Part model, mm, in its own coordinate system. Face numbers are marked on the shaded views. Round coordinates to 2 decimals unless told otherwise and drop trailing zeros. Order: outer loops, then holes, each group sorted by start corner. A loop starts at its lowest first (then second) coordinate and runs counter-clockwise, first axis right, second up. Notation, with made-up numbers: (-31.5, 54) - (12.5, 54) arc R16 cw to (12.5, 69) - close; hole circle Ø2 at (-9.75, 47.25). An arc over 180 degrees is marked (long way). Return JSON: item names as keys, results as strings. Group by question number.
Item 1: Saw through at D-D on x = 14.5. List the corners of the cut face in (y, z), and give its area (3 significant figures).
Item 2: Drop flat-ended pins along their axis: pin 1 (6.5 mm diameter, centred on x = 5.5, z = 80.5, fed in from +Y) (3 decimals); pin 2 (1 mm diameter, centred on x = 21, z = 222, fed in from +Y); pin 3 (11 mm diameter, centred on x = 26, y = 218.5, fed in from +Z); pin 4 (22 mm diameter, centred on y = 193.5, z = 265, fed in from +X). Give the stop position or say it passes through.
Item 3: Two-plate mould, pull along X, no slides. Class the marked faces 1, 2 and 3: released by +X, released by -X, zero draft, split by the parting line, or undercut.
Item 4: Probe probe 1 along Z at (x, y) = (12.5, 105.5); probe 2 along Y at (x, z) = (16, 85); probe 3 along Y at (x, z) = (17, 51). List the from-to ranges inside material, lowest first.
```python
from build123d import *

# Parameters (mm, degrees)
BOSS_EXTRUDE3_DEPTH     = 10
BOSS_EXTRUDE4_DEPTH     = 30
CUT_EXTRUDE1_DEPTH      = 10
CUT_EXTRUDE1_DEPTH_BACK = 1
FILLET1_R               = 10
BOSS_EXTRUDE5_DEPTH     = 21
CUT_EXTRUDE2_DEPTH      = 21
FILLET2_R               = 10
SKETCH15_R              = 3
CUT_EXTRUDE3_DEPTH      = 21
SKETCH16_R              = 22
CUT_EXTRUDE4_DEPTH      = 10


with BuildPart() as part:
    # Sketch1 → Boss-Extrude3 (new body)
    with BuildSketch(Plane(origin=(0, 0, 0), x_dir=(0, 0, -1), z_dir=(1, 0, 0))):
        with BuildLine():
            Line((-20, 0), (-20, 300))
            ThreePointArc((-20, 300), (0, 320), (20, 300))
            Line((20, 300), (20, 0))
            ThreePointArc((20, 0), (0, -20), (-20, 0))
        make_face()
    extrude(amount=BOSS_EXTRUDE3_DEPTH)

    # Sketch1<5> → Boss-Extrude4 (add)
    with BuildSketch(Plane(origin=(0, 0, 0), x_dir=(0, 0, -1), z_dir=(1, 0, 0))):
        with BuildLine():
            Line((-30, 300), (-30, 0))
            ThreePointArc((-30, 0), (0, -30), (30, 0))
            Line((30, 0), (30, 300))
            ThreePointArc((30, 300), (0, 330), (-30, 300))
        make_face()
        with BuildLine():
            Line((-20, 0), (-20, 300))
            ThreePointArc((-20, 300), (0, 320), (20, 300))
            Line((20, 300), (20, 0))
            ThreePointArc((20, 0), (0, -20), (-20, 0))
        make_face(mode=Mode.SUBTRACT)
    extrude(amount=BOSS_EXTRUDE4_DEPTH)

    # Sketch2 → Cut-Extrude1 (cut, two sides: drawn at the far end of the back side and taken through both)
    with BuildSketch(Plane(origin=(10, 0, 0), x_dir=(0, 0, -1), z_dir=(1, 0, 0)).offset(-CUT_EXTRUDE1_DEPTH_BACK)):
        with BuildLine():
            Line((-25, 0), (-25, 300))
            ThreePointArc((-25, 300), (0, 325), (25, 300))
            Line((25, 300), (25, 0))
            ThreePointArc((25, 0), (0, -25), (-25, 0))
        make_face()
    extrude(amount=CUT_EXTRUDE1_DEPTH + CUT_EXTRUDE1_DEPTH_BACK, mode=Mode.SUBTRACT)

    # Fillet1
    fillet1_edges = [part.edges().sort_by_distance(p)[0] for p in [
        (30, 330, 0),
        (30, 150, 30),
        (30, -30, 0),
        (30, 150, -30),
    ]]
    fillet(fillet1_edges, radius=FILLET1_R - 0.0001)  # a hair under: the kernel refuses the full size

    # Sketch4 → Boss-Extrude5 (add)
    with BuildSketch(Plane.ZY.offset(-20)):
        with BuildLine():
            Line((30, 300), (30, 150))
            Line((30, 150), (330, 150))
            Line((330, 150), (330, 190))
            Line((330, 190), (300.476136934, 195.7258523))
            ThreePointArc((300.476136934, 195.7258523), (276.739397408, 219.4512428), (245.854526043, 206.319156964))
            Line((245.854526043, 206.319156964), (225.44540351, 210.277298245))
            Line((225.44540351, 210.277298245), (209.44540351, 210.277298245))
            Line((209.44540351, 210.277298245), (30, 300))
        make_face()
    extrude(amount=BOSS_EXTRUDE5_DEPTH)

    # Sketch6 → Cut-Extrude2 (cut)
    with BuildSketch(Plane(origin=(20, 0, 0), x_dir=(0, 0, -1), z_dir=(1, 0, 0))):
        Polygon((-40, 160), (-40, 213.989666216), (-172.534869505, 174.229205364), (-172.534869505, 160), align=None)
        Polygon((-40, 283.819660113), (-172.534869505, 217.55222536), (-172.534869505, 187.801603826), (-40, 227.562064677), align=None)
    extrude(amount=-CUT_EXTRUDE2_DEPTH, mode=Mode.SUBTRACT)

    # Fillet2
    fillet2_edges = [part.edges().sort_by_distance(p)[0] for p in [
        (9.5, 190, 330),
    ]]
    fillet(fillet2_edges, radius=FILLET2_R)

    # Sketch15 → Cut-Extrude3 (cut)
    with BuildSketch(Plane.ZY.offset(1)):
        with Locations((270.877121852, 189.785242032)):
            Circle(SKETCH15_R)
    extrude(amount=-CUT_EXTRUDE3_DEPTH, mode=Mode.SUBTRACT)

    # Sketch16 → Cut-Extrude4 (cut)
    with BuildSketch(Plane(origin=(20, 0, 0), x_dir=(0, 0, -1), z_dir=(1, 0, 0))):
        with Locations((-270.877121852, 189.785242032)):
            Circle(SKETCH16_R)
    extrude(amount=-CUT_EXTRUDE4_DEPTH, mode=Mode.SUBTRACT)


solid = part.part
```
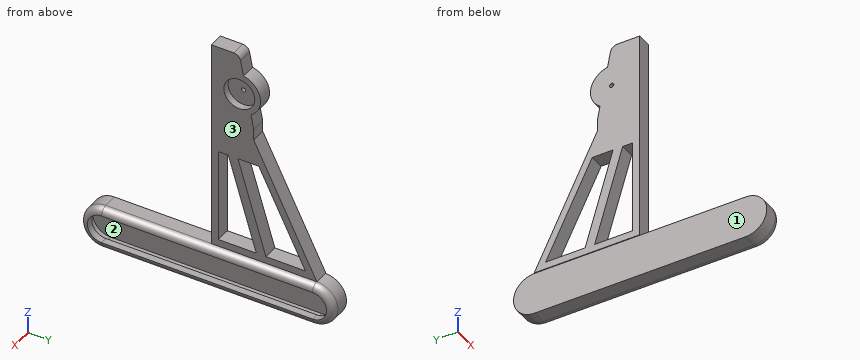
Filled in:
{
 "1": {"outline": "(0, -30) - (300, -30) arc R30 ccw to (300, 30) - (210.28, 209.45) - (210.28, 225.45) - (206.32, 245.85) arc R30 ccw to (195.73, 300.48) - (191.57, 321.9) arc R10 ccw to (181.75, 330) - (150, 330) - (150, 30) - (0, 30) arc R30 ccw to start; hole (0, -25) - (300, -25) arc R25 ccw to (300, 25) - (0, 25) arc R25 ccw to start; hole (160, 40) - (213.99, 40) - (174.23, 172.53) - (160, 172.53) - close; hole circle Ø44 at (189.79, 270.88); hole (187.8, 172.53) - (227.56, 40) - (283.82, 40) - (217.55, 172.53) - close", "area": "17,900 mm^2"},
 "2": {"pin 1": "stops at y = 276.375", "pin 2": "passes through", "pin 3": "stops at z = 29.99", "pin 4": "stops at x = 10"},
 "3": {"face 1": "released by -X", "face 2": "undercut", "face 3": "released by +X"},
 "4": {"probe 1": "z = -30 to -25, 25 to 30", "probe 2": "y = 150 to 160, 200.49 to 214.06, 261.32 to 272.5", "probe 3": "y = 150 to 160, 210.69 to 224.26, 278.32 to 289.5"}
}
